```python
from build123d import *

# Parameters (mm, degrees)
F2_R     = 250
F3_R     = 20
F4_R     = 15.5
F5_DEPTH = 25


with BuildPart() as f1:
    # F0 (on Right) → F1 (revolve)
    with BuildSketch(Plane.YZ):
        Polygon((0, 533.4), (0, 200), (10, 200), (10, 533.4), (610, 533.4), (610, 983.4), (-290, 983.4), (-290, 533.4), align=None)
    revolve(axis=Axis((0, 333.333626, 0), (0, 1, 0)))

    # F2
    f2_edges = [f1.edges().sort_by_distance(p)[0] for p in [
        (0, -290, -983.4),
        (0, 610, -983.4),
    ]]
    fillet(f2_edges, radius=F2_R)

    # F3
    f3_edges = [f1.edges().sort_by_distance(p)[0] for p in [
        (0, -290, -533.4),
        (0, 610, -533.4),
    ]]
    fillet(f3_edges, radius=F3_R)

    # F4 (on face) → F5 (cut)
    with BuildSketch(Plane.XZ):
        with Locations((0, 240)):
            Circle(F4_R)
        with Locations((-169.705627, 169.705627)):
            Circle(F4_R)
        with Locations((-240, 0)):
            Circle(F4_R)
        with Locations((-169.705627, -169.705627)):
            Circle(F4_R)
        with Locations((0, -240)):
            Circle(F4_R)
        with Locations((169.705627, -169.705627)):
            Circle(F4_R)
        with Locations((240, 0)):
            Circle(F4_R)
        with Locations((169.705627, 169.705627)):
            Circle(F4_R)
    extrude(amount=-F5_DEPTH, mode=Mode.SUBTRACT)


solid = f1.part
```
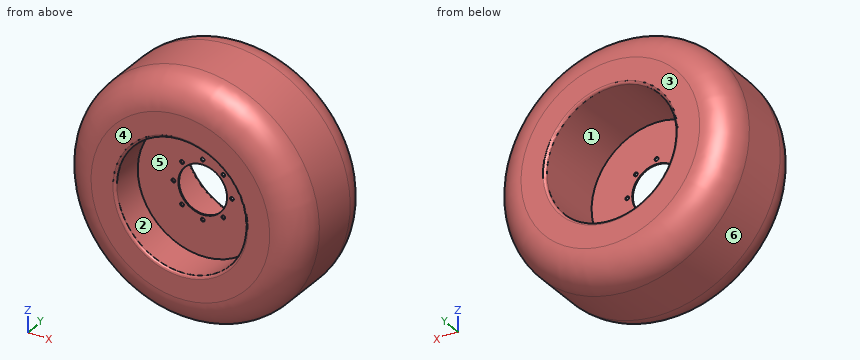
Source: CAD feature listing. Evaluate the final solid. Frame: model axes, mm. Face numbers are marked on the shaded views. A direction names the side the tool comes from. Coordinates: 2 decimals unless noted, no trailing zeros. Write each loop counter-clockwise with the first axis right and the second up, starting at its lowest first coordinate (ties: lowest second). Pieces come first, ordered by that corner, then holes. Notation, with made-up numbers: (42.25, 80) - (48.25, 80) arc R19 cw to (48.25, 104) - close; hole circle Ø1 at (65.5, 81.25). An arc over 180 degrees is marked (long way). Answer as a JSON object with one key per item and string values.
Q1. Set-up query: the marked faces 1, 2 and 3. Return all of +Z, -Z, +X, -X, +Y, -Y with unobstructed straight access to the full face (end or side cutting, diameter ignored); none if empty.
Ans:
{"face 1": "+Y", "face 2": "-Y", "face 3": "+Z, -Z, +X, -X, +Y"}
Q2. Draft query along X for the marked faces 4, 5 and 6. Return one class per face: released by +X, released by -X, zero draft, split by the parting line, or undercut.
Ans:
{"face 4": "zero draft", "face 5": "undercut", "face 6": "split by the parting line"}
Q3. First-contact query: pin 1 Ø5 at (x, z) = (355, 18) entering from +Y; pin 2 Ø2 at (x, y) = (-330, 232.5) entering from -Z; pin 3 Ø5 at (y, z) = (-118.5, -98.5) entering from +X. Flat tips, straight axial feed; report the tip coordinate or a pass-through.
Ans:
{"pin 1": "stops at y = 10", "pin 2": "stops at z = -926.73", "pin 3": "stops at x = 966.6"}
Q4. Section query A-A, the plane y = 320. Output: boundary loops of the cut face in (x, z).
Ans:
{"outline": "circle Ø1966.8 at (0, 0); hole circle Ø1066.8 at (0, 0)"}
Q5. Section query B-B, the plane y = -83. Output: boundary loops of the cut face in (x, z), plus the area to 3 significant figures.
Ans:
{"outline": "circle Ø1959.35 at (0, 0); hole circle Ø1066.8 at (0, 0)", "area": "2,120,000 mm2"}
Q6. Material intervals for line 1 (Y direction, x = 268, z = 250); line 2 (X direction, y = -253, z = -11); line 3 (X direction, y = 497.5, z = -130), sorted ascending. Write a range as [from, to].
Ans:
{"line 1": "y = [0, 10]", "line 2": "x = [-864.22, -533.29], [533.29, 864.22]", "line 3": "x = [-933.18, -517.32], [517.32, 933.18]"}
